Geometry check sheet. Reference: the model listing, model coordinates, mm. Face numbers are marked on the shaded views. A direction names the side the tool comes from. Give positions to 0.01 mm unless a question says otherwise; leave off trailing zeros. Loops run counter-clockwise (first coordinate to the right, second up) from the corner with the lowest first, then second, coordinate; pieces in that order, holes last.
1. Cross-section at A-A, the plane x = 0. Record the cut outline in (y, z).
2. Tool access check on the marked faces 4 and 5. Record the directions out of +Z, -Z, +X, -X, +Y, -Y that give a thin tool (end or side, any length) a straight path to the whole face; none if there is none.
3. Go/stop test with flat-tipped pins: pin 1 Ø3 at (x, z) = (-21, -10) entering from -Y; pin 2 Ø12 at (x, y) = (-18.5, -15.5) entering from +Z; pin 3 Ø4 at (x, y) = (-18, -25) entering from -Z (3 decimals); pin 4 Ø14 at (x, y) = (0, 0) entering from -Z (3 decimals). Record where each tip stops, or that it passes through.
4. Release check for a two-part mould opening along Y. For the marked faces 1, 2 and 3 record: +Y half, -Y half, draft (parallel to the pull), parting line (faces both ways), or undercut.
5. Cross-section at D-D, the plane z = -30.5. Record the cut outline in (x, y).
6. Cross-section at B-B, the plane z = -4.5. Record the cut outline in (x, y), plus the area to 3 significant figures.
7. Material ranges on L1, parallel to Y at x = 0, z = -35.5; L2, parallel to X at y = 15.5, z = -12, recorded low to high.
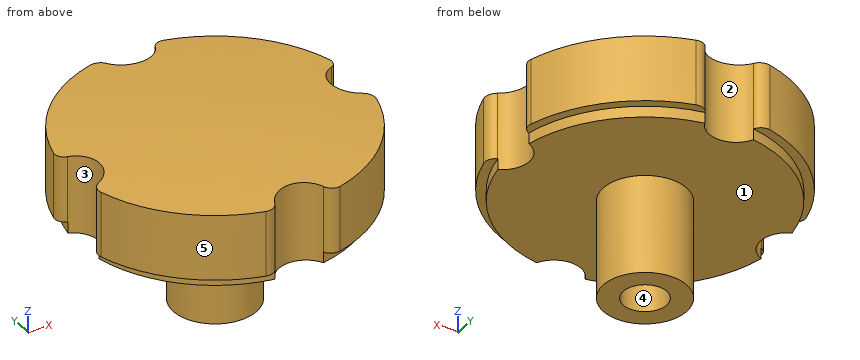
from build123d import *

# Parameters (mm, degrees)
CUT_EXTRUDE1_REACH = 77.502
SKETCH2_R          = 7.5
FILLET1_R          = 3


with BuildPart() as part:
    # Sketch1 → Revolve1 (revolve)
    with BuildSketch(Plane(origin=(0, 0, 0), x_dir=(1, 0, 0), z_dir=(0, 1, 0))):
        with BuildLine():
            Line((0, 20.005025157), (0, 0))
            ThreePointArc((0, 0), (-20.025110024, 0.501570756), (-40, 2.005025157))
            Line((-40, 2.005025157), (-40, 20.005025157))
            Line((-40, 20.005025157), (-37.5, 20.005025157))
            Line((-37.5, 20.005025157), (-37.5, 23.005025157))
            Line((-37.5, 23.005025157), (-11.5, 23.005025157))
            Line((-11.5, 23.005025157), (-11.5, 50.005025157))
            Line((-11.5, 50.005025157), (-6, 50.005025157))
            Line((-6, 50.005025157), (-6, 20.005025157))
            Line((-6, 20.005025157), (0, 20.005025157))
        make_face()
    revolve(axis=Axis((0, 0, -358.843484937), (0, 0, 1)))

    # Sketch2 → Cut-Extrude1 (cut, up to next)
    with BuildSketch(Plane.XY, mode=Mode.PRIVATE) as cut_extrude1_sk1:
        with Locations((0, 40)):
            Circle(SKETCH2_R)
    cut_extrude1_tool1 = extrude(cut_extrude1_sk1.sketch, amount=-CUT_EXTRUDE1_REACH, mode=Mode.PRIVATE) & part.part
    # Sketch2 → Cut-Extrude1 (cut, up to next)
    with BuildSketch(Plane.XY, mode=Mode.PRIVATE) as cut_extrude1_sk2:
        with Locations((40, 0)):
            Circle(SKETCH2_R)
    cut_extrude1_tool2 = extrude(cut_extrude1_sk2.sketch, amount=-CUT_EXTRUDE1_REACH, mode=Mode.PRIVATE) & part.part
    # Sketch2 → Cut-Extrude1 (cut, up to next)
    with BuildSketch(Plane.XY, mode=Mode.PRIVATE) as cut_extrude1_sk3:
        with Locations((0, -40)):
            Circle(SKETCH2_R)
    cut_extrude1_tool3 = extrude(cut_extrude1_sk3.sketch, amount=-CUT_EXTRUDE1_REACH, mode=Mode.PRIVATE) & part.part
    # Sketch2 → Cut-Extrude1 (cut, up to next)
    with BuildSketch(Plane.XY, mode=Mode.PRIVATE) as cut_extrude1_sk4:
        with Locations((-40, 0)):
            Circle(SKETCH2_R)
    cut_extrude1_tool4 = extrude(cut_extrude1_sk4.sketch, amount=-CUT_EXTRUDE1_REACH, mode=Mode.PRIVATE) & part.part
    add(cut_extrude1_tool1.solids().sort_by_distance((0, 40, 0))[0], mode=Mode.SUBTRACT)
    add(cut_extrude1_tool2.solids().sort_by_distance((40, 0, 0))[0], mode=Mode.SUBTRACT)
    add(cut_extrude1_tool3.solids().sort_by_distance((0, -40, 0))[0], mode=Mode.SUBTRACT)
    add(cut_extrude1_tool4.solids().sort_by_distance((-40, 0, 0))[0], mode=Mode.SUBTRACT)

    # Fillet1
    # the kernel refuses this fillet: 3 mm, written as the material it takes off along each edge
    with BuildSketch(Plane(origin=(-39.296875, -7.466968276, -27.456580588), x_dir=(0.9673809008255011, 0.25332625745872106, 0), z_dir=(0, 0, 1))) as fillet1_piece_1:
        with BuildLine():
            CenterArc((2.907334637, -2.960609009), FILLET1_R, 99.295051663, 81.059690814)
            ThreePointArc((-0.092607863, -2.979183163), (-0.074063004, -1.488728691), (0, 0))
            ThreePointArc((0, 0), (1.211389432, -0.098477478), (2.422778864, 0))
        make_face()
    extrude(amount=32.903111461, mode=Mode.SUBTRACT)
    with BuildSketch(Plane(origin=(-39.296875, 7.466968276, -27.456580588), x_dir=(0.967380900825501, -0.25332625745872067, 0), z_dir=(0, 0, 1))) as fillet1_piece_2:
        with BuildLine():
            CenterArc((2.907334637, 2.960609009), FILLET1_R, 179.645257523, 81.059690814)
            ThreePointArc((-0.092607863, 2.979183163), (-0.074063004, 1.488728691), (0, 0))
            ThreePointArc((0, 0), (1.211389432, 0.098477478), (2.422778864, 0))
        make_face()
    extrude(amount=32.903110861, mode=Mode.SUBTRACT)
    with BuildSketch(Plane(origin=(7.466968276, -39.296875, -27.456580588), x_dir=(-0.2533262574587217, 0.9673809008255008, 0), z_dir=(0, 0, 1)), Plane(origin=(39.296875, 7.466968276, -27.456580588), x_dir=(-0.9673809008255009, -0.25332625745872134, 0), z_dir=(0, 0, 1)), Plane(origin=(-7.466968276, 39.296875, -27.456580588), x_dir=(0.2533262574587217, -0.9673809008255008, 0), z_dir=(0, 0, 1))) as fillet1_piece_3:
        with BuildLine():
            CenterArc((2.907334637, -2.960609009), FILLET1_R, 99.295051663, 81.059690814)
            ThreePointArc((-0.092607863, -2.979183163), (-0.074063004, -1.488728691), (0, 0))
            ThreePointArc((0, 0), (1.211389432, -0.098477478), (2.422778864, 0))
        make_face()
    extrude(amount=32.903110861, mode=Mode.SUBTRACT)
    with BuildSketch(Plane(origin=(-7.466968276, -39.296875, -27.456580588), x_dir=(-0.974784701688693, 0.22314745204390218, 0), z_dir=(0, 0, 1)), Plane(origin=(39.296875, -7.466968276, -27.456580588), x_dir=(-0.2231474520439016, -0.9747847016886931, 0), z_dir=(0, 0, 1)), Plane(origin=(7.466968276, 39.296875, -27.456580588), x_dir=(0.9747847016886936, -0.22314745204390027, 0), z_dir=(0, 0, 1))) as fillet1_piece_4:
        with BuildLine():
            CenterArc((2.868848841, -2.997917064), FILLET1_R, 87.864792425, 81.059690814)
            ThreePointArc((-0.075275684, -2.421609175), (0.060792092, -1.21386428), (0, 0))
            ThreePointArc((0, 0), (1.490311086, 0.027772481), (2.980622172, 0))
        make_face()
    extrude(amount=32.903110861, mode=Mode.SUBTRACT)


solid = part.part
Result:
1. outline: (-32.5, -23.01) - (-11.5, -23.01) - (-11.5, -50.01) - (-6, -50.01) - (-6, -20.01) - (6, -20.01) - (6, -50.01) - (11.5, -50.01) - (11.5, -23.01) - (32.5, -23.01) - (32.5, -1.32) arc R400 ccw to (-32.5, -1.32) - close
2. face 4: -Z
2. face 5: +Z, -Z, -X, -Y
3. pin 1: stops at y = -34.92
3. pin 2: stops at z = -0.41
3. pin 3: stops at z = -23.005
3. pin 4: stops at z = -50.005
4. face 1: draft
4. face 2: +Y half
4. face 3: undercut
5. outline: circle Ø23 at (0, 0); hole circle Ø12 at (0, 0)
6. outline: (-38.63, -10.37) arc R40 ccw to (-10.37, -38.63) arc R3 ccw to (-6.85, -36.95) arc R7.5 cw to (6.85, -36.95) arc R3 ccw to (10.37, -38.63) arc R40 ccw to (38.63, -10.37) arc R3 ccw to (36.95, -6.85) arc R7.5 cw to (36.95, 6.85) arc R3 ccw to (38.63, 10.37) arc R40 ccw to (10.37, 38.63) arc R3 ccw to (6.85, 36.95) arc R7.5 cw to (-6.85, 36.95) arc R3 ccw to (-10.37, 38.63) arc R40 ccw to (-38.63, 10.37) arc R3 ccw to (-36.95, 6.85) arc R7.5 cw to (-36.95, -6.85) arc R3 ccw to start
6. area: 4,670 mm2
7. L1: y = -11.5 to -6, 6 to 11.5
7. L2: x = -36.87 to 36.87
